```python
from build123d import *

# Parameters (mm, degrees)
F0_W     = 508
F0_H     = 1016
F1_DEPTH = 508
F2_R     = 63.5
F3_DEPTH = 508.001
F4_R     = 63.5
F5_SIZE  = 127


with BuildPart() as f1:
    # F0 (on Front) → F1 (new body)
    with BuildSketch(Plane.XZ):
        Rectangle(F0_W, F0_H)
    extrude(amount=F1_DEPTH)

    # F2 (on face) → F3 (cut, through all)
    with BuildSketch(Plane.XZ.offset(508)):
        Circle(F2_R)
    extrude(amount=-F3_DEPTH, mode=Mode.SUBTRACT)

    # F4
    f4_edges = [f1.edges().sort_by_distance(p)[0] for p in [
        (254, -254, 508),
        (-254, -254, 508),
    ]]
    fillet(f4_edges, radius=F4_R)

    # F5
    f5_edges = [f1.edges().sort_by_distance(p)[0] for p in [
        (254, -254, -508),
        (-254, -254, -508),
    ]]
    chamfer(f5_edges, length=F5_SIZE)


solid = f1.part
```
Check sheet for the modelled part. Datum: model origin and axes. Units: mm. Round coordinates to 2 decimals unless told otherwise and drop trailing zeros. Loops run counter-clockwise (first coordinate to the right, second up) from the corner with the lowest first, then second, coordinate; pieces in that order, holes last. Notation, with made-up numbers: (69, -37) -> (79, -37) arc R22 ccw to (79, -18) -> close; hole circle Ø11 at (-38.75, -28.5). An arc over 180 degrees is marked (long way). Answer in a Markdown table with one row per item.
Q1. Sectioned sample at B-B on x = 0. Enter the section's corners in (y, z), then the cut area to 3 significant figures.
Data:
| item | result |
|---|---|
| outline | (-508, -508) -> (0, -508) -> (0, -63.5) -> (-508, -63.5) -> close; (-508, 63.5) -> (0, 63.5) -> (0, 508) -> (-508, 508) -> close |
| area | 452,000 mm^2 |
Q2. Sectioned sample at A-A on y = -282. Enter the section's corners in (x, z).
Data:
| item | result |
|---|---|
| outline | (-254, -381) -> (-127, -508) -> (127, -508) -> (254, -381) -> (254, 444.5) arc R63.5 ccw to (190.5, 508) -> (-190.5, 508) arc R63.5 ccw to (-254, 444.5) -> close; hole circle Ø127 at (0, 0) |
Q3. Go/stop test with flat-tipped pins: P1, Ø12, axis at x = -202, y = -59, coming from the +Z side; P2, Ø2, axis at y = -367.5, z = -403, coming from the -X side. Record where each tip stops, or that it passes through.
Data:
| item | result |
|---|---|
| P1 | stops at z = 507.76 |
| P2 | stops at x = -233 |
Q4. Thickness scan on L1, parallel to Z at x = 0, y = -119; L2, parallel to Z at x = -11.5, y = -305; L3, parallel to Z at x = -135, y = -476. Record the ranges inside material, lowest first.
Data:
| item | result |
|---|---|
| L1 | z = -508 to -63.5, 63.5 to 508 |
| L2 | z = -508 to -62.45, 62.45 to 508 |
| L3 | z = -500 to 508 |
Q5. Release check for a two-part mould opening along Z. For faces 1 (the face through (-13.77, -257.56, -61.99)), 2 (the face through (234.905, -257.556, 489.892)), 3 (the face through (-4, 0, 120)), 4 (the face through (-2, -250, -508)) record: released by +Z, released by -Z, zero draft, split by the parting line, or undercut.
Data:
| item | result |
|---|---|
| face 1 | undercut |
| face 2 | released by +Z |
| face 3 | zero draft |
| face 4 | released by -Z |
Q6. Sectioned sample at C-C on z = 0. Enter the section's corners in (x, y), then the cut area to 3 significant figures.
Data:
| item | result |
|---|---|
| outline | (-254, -508) -> (-63.5, -508) -> (-63.5, 0) -> (-254, 0) -> close; (63.5, -508) -> (254, -508) -> (254, 0) -> (63.5, 0) -> close |
| area | 194,000 mm^2 |
